Work out the finished part from the listing and answer in its coordinate system (mm). Face numbers are marked on the shaded views. A direction names the side the tool comes from. Coordinates: 2 decimals unless noted, no trailing zeros. Write each loop counter-clockwise with the first axis right and the second up, starting at its lowest first coordinate (ties: lowest second). Pieces come first, ordered by that corner, then holes. Notation, with made-up numbers: M 52,63.5 L 103,63.5 A17 ccw 103,86.5 Z; hole C 44,32.5 d3. An arc over 180 degrees is marked long. Answer as CSV lines item,"result". Start each with the question number.
(1) A cutting plane is placed at B-B on x = 0. Give the vertices of the cut face in (y, z).
(2) For the marked faces 1 and 2, determine the directions among +Z, -Z, +X, -X, +Y, -Y from which every point of the face is accessible in a straight line to the end or side of a thin tool.
(3) Flat-ended cylindrical pins translate along their axes: P1, Ø1.5, axis at x = -10, z = 10, coming from the +Y side; P2, Ø3, axis at x = 37.5, y = 23.5, coming from the +Z side; P3, Ø5, axis at x = 27.5, z = -34, coming from the +Y side; P4, Ø16, axis at x = -25, z = 80, coming from the +Y side. Find the tip coordinate at first contact, or state that the pin passes through.
(4) A cutting plane is placed at C-C on y = 61. Give the vertices of the cut face in (x, z).
(5) A cutting plane is placed at A-A on z = -21. Give the vertices of the cut face in (x, y).
(6) A cutting plane is placed at D-D on z = -82. Give the vertices of the cut face in (x, y), then the cut area to 3 significant figures.
(7) Find the intervals of material crossed by L1, parallel to Z at x = -25, y = 7; L2, parallel to X at y = 4, z = -32.5; L3, parallel to Y at x = -1.5, z = 50, in increasing order. Write a range as [from, to].
from build123d import *

# Parameters (mm, degrees)
BOSS_EXTRUDE1_DEPTH      = 50
BOSS_EXTRUDE1_DEPTH_BACK = 50
CHAMFER1_SIZE            = 20
HOLE1_D                  = 10
CUT_EXTRUDE1_DEPTH       = 125.599357944
SKETCH7_W                = 100
SKETCH7_H                = 55
CUT_EXTRUDE2_DEPTH       = 206.243757518
BOSS_EXTRUDE2_DEPTH      = 20
HOLE2_D                  = 20


with BuildPart() as part:
    # Sketch1 → Boss-Extrude1 (new, two sides: drawn at the far end of the back side and taken through both)
    with BuildSketch(Plane(origin=(0, 0, 0), x_dir=(0, 0, -1), z_dir=(1, 0, 0)).offset(-BOSS_EXTRUDE1_DEPTH_BACK)):
        Polygon((-100, 0), (100, 0), (100, 85), (80, 85), (80, 30), (-20, 30), (-20, 10), (-100, 10), align=None)
    extrude(amount=BOSS_EXTRUDE1_DEPTH + BOSS_EXTRUDE1_DEPTH_BACK)

    # Chamfer1
    chamfer1_edges = [part.edges().sort_by_distance(p)[0] for p in [
        (50, 5, 100),
        (-50, 5, 100),
    ]]
    chamfer(chamfer1_edges, length=CHAMFER1_SIZE)

    # Hole1 (through all)
    with Locations(Plane(origin=(0, 10, 0), x_dir=(1, 0, 0), z_dir=(0, 1, 0))):
        with Locations((-25, -40), (-25, -80)):
            hole1 = Hole(HOLE1_D / 2)

    # Mirror1: Hole1 across plane
    add(hole1.mirror(Plane(origin=(0, 0, 0), x_dir=(0, 0, 1), z_dir=(1, 0, 0))), mode=Mode.SUBTRACT)

    # Sketch4 → Cut-Extrude1 (cut, through all)
    with BuildSketch(Plane(origin=(0, 30, 0), x_dir=(1, 0, 0), z_dir=(0, 1, 0))):
        with BuildLine():
            Line((-19, 50), (-19, 0))
            ThreePointArc((-19, 0), (-25, -6), (-31, 0))
            Line((-31, 0), (-31, 50))
            ThreePointArc((-31, 50), (-25, 56), (-19, 50))
        make_face()
        with BuildLine():
            Line((19, 50), (19, 0))
            ThreePointArc((19, 0), (25, -6), (31, 0))
            Line((31, 0), (31, 50))
            ThreePointArc((31, 50), (25, 56), (19, 50))
        make_face()
    extrude(amount=-CUT_EXTRUDE1_DEPTH, mode=Mode.SUBTRACT)

    # Sketch7 → Cut-Extrude2 (cut, through all)
    with BuildSketch(Plane.XY.offset(-80)):
        with Locations((0, 57.5)):
            Rectangle(SKETCH7_W, SKETCH7_H)
    extrude(amount=-CUT_EXTRUDE2_DEPTH, mode=Mode.SUBTRACT)

    # Sketch8 → Boss-Extrude2 (add)
    with BuildSketch(Plane(origin=(0, 0, -100), x_dir=(-1, 0, 0), z_dir=(0, 0, -1))):
        with BuildLine():
            Line((50, 30), (-50, 30))
            Line((-50, 30), (-19.867631849, 74.463922337))
            ThreePointArc((-19.867631849, 74.463922337), (0, 85), (19.867631849, 74.463922337))
            Line((19.867631849, 74.463922337), (50, 30))
        make_face()
    extrude(amount=-BOSS_EXTRUDE2_DEPTH)

    # Hole2 (through all)
    with Locations(Plane.XY.offset(-80)):
        with Locations((0, 61)):
            Hole(HOLE2_D / 2)


solid = part.part
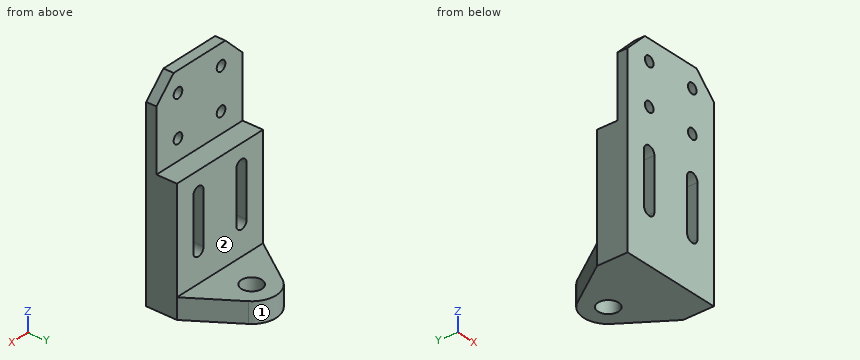
Here are the results:
1,outline,"M 0,-100 L 51,-100 L 51,-80 L 30,-80 L 30,20 L 10,20 L 10,100 L 0,100 Z; M 71,-100 L 85,-100 L 85,-80 L 71,-80 Z"
2,face 1,"+Z, -Z, +Y"
2,face 2,"+Z, +X, -X, +Y"
3,P1,"stops at y = 30"
3,P2,"stops at z = 20"
3,P3,"passes through"
3,P4,"stops at y = 10"
4,outline,"M -28.99,-100 L -10,-100 L -10,-80 L -28.99,-80 Z; M 10,-100 L 28.99,-100 L 28.99,-80 L 10,-80 Z"
5,outline,"M -50,0 L -31,0 L -31,30 L -50,30 Z; M -19,0 L 19,0 L 19,30 L -19,30 Z; M 31,0 L 50,0 L 50,30 L 31,30 Z"
6,outline,"M -50,0 L 50,0 L 50,30 L 19.87,74.46 A24 ccw -19.87,74.46 L -50,30 Z; hole C 0,61 d20"
6,area,"6,090 mm^2"
7,L1,"z = [-100, -56], [6, 35], [45, 75], [85, 100]"
7,L2,"x = [-50, -31], [-19, 19], [31, 50]"
7,L3,"y = [0, 10]"
